Source: three-view drawing plus pictorial views. Frame: mm from the lowest corner of the part. A direction names the side the tool comes from. Coordinates: 2 decimals unless noted, no trailing zeros. Write each loop counter-clockwise with the first axis right and the second up, starting at its lowest first coordinate (ties: lowest second). Pieces come first, ordered by that corner, then holes. Notation, with made-up numbers: M 43,52 L 58,52 A34 ccw 58,84 Z; hole C 46,62 d10. An arc over 180 degrees is marked long. Write item = value, one per line. Start each with the question number.
Item 1: Ray query, L1, parallel to X at y = 1, z = 19; L2, parallel to Y at x = 18, z = 0.85; L3, parallel to X at y = 37.5, z = 2.8 (1 decimal). Return the intervals inside material, ascending. Write a range as [from, to].
Item 2: Section A-A on z = 19. Output: boundary loops of the cut face in (x, y).
Item 3: First-contact query: pin 1 Ø10 at (y, z) = (39, 7.5) entering from -X; pin 2 Ø5 at (x, y) = (18, 15) entering from +Z; pin 3 Ø8 at (x, z) = (30, 26) entering from +Y. Flat tips, straight axial feed; report the tip coordinate or a pass-through.
Item 4: Section B-B on y = 15. Output: boundary loops of the cut face in (x, z), plus the area to 3 significant figures.
Item 5: Section D-D on x = 23.5. Output: boundary loops of the cut face in (y, z), plus the area to 3 significant figures.
Item 6: Section C-C on x = 18. Output: boundary loops of the cut face in (y, z).
Item 7: Pull-direction query (X, two-part tool) for the marked faces 3, 4 and 5; classes: +X half, -X half, draft (parallel to the pull), parting line (faces both ways), or undercut.
Item 8: Reachability of the marked faces 1 and 2 from +Z, -Z, +X, -X, +Y, -Y: full face, straight path, thin tool, end or side. Return the list, or none.
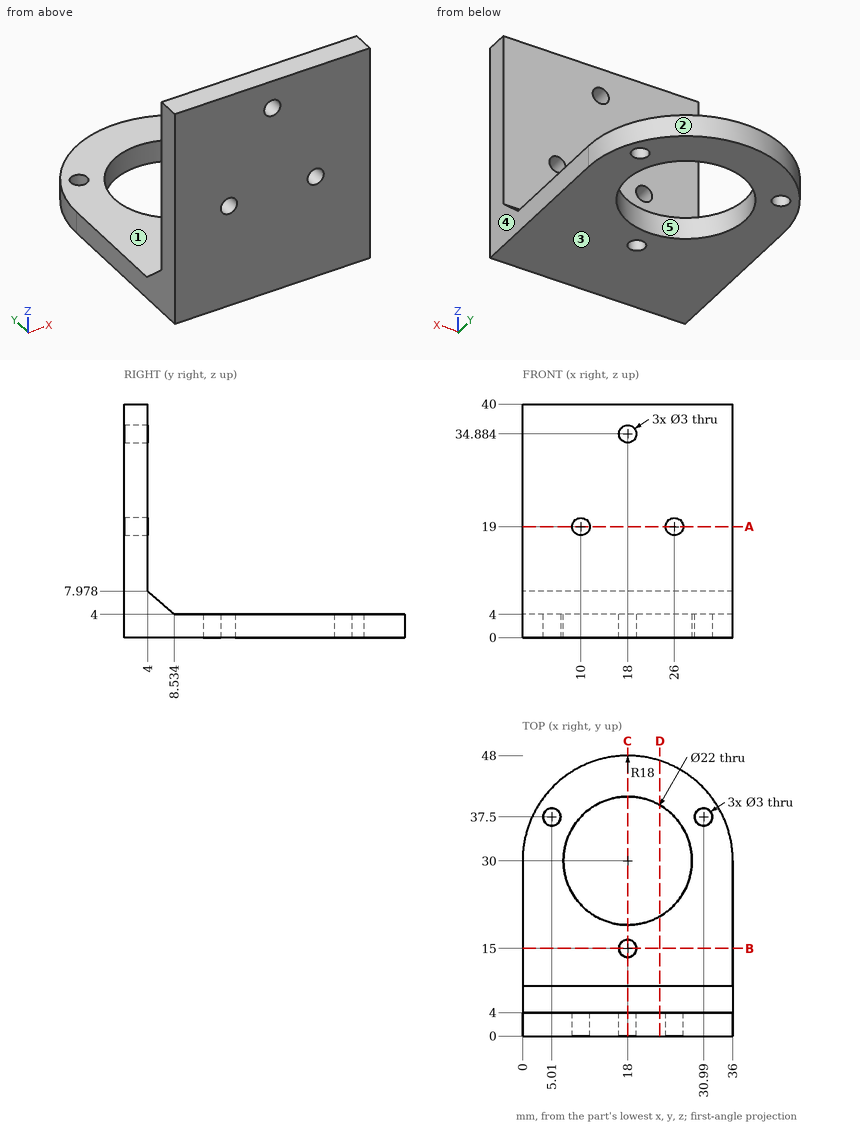
Responses:
q1.L1 = [0, 8.5], [11.5, 24.5], [27.5, 36]
q1.L2 = [0, 13.5], [16.5, 19], [41, 48]
q1.L3 = [1.6, 3.5], [6.5, 10], [26, 29.5], [32.5, 34.4]
q2.outline = M 0,0 L 8.5,0 L 8.5,4 L 0,4 Z; M 11.5,0 L 24.5,0 L 24.5,4 L 11.5,4 Z; M 27.5,0 L 36,0 L 36,4 L 27.5,4 Z
q3.pin_1 = 0.84
q3.pin_2 = 4
q3.pin_3 = 4
q4.outline = M 0,0 L 16.5,0 L 16.5,4 L 0,4 Z; M 19.5,0 L 36,0 L 36,4 L 19.5,4 Z
q4.area = 132 mm²
q5.outline = M 0,0 L 20.47,0 L 20.47,4 L 8.53,4 L 4,7.98 L 4,40 L 0,40 Z; M 39.53,0 L 47.14,0 L 47.14,4 L 39.53,4 Z
q5.area = 265 mm²
q6.outline = M 0,0 L 13.5,0 L 13.5,4 L 8.53,4 L 4,7.98 L 4,33.38 L 0,33.38 Z; M 0,36.38 L 4,36.38 L 4,40 L 0,40 Z; M 16.5,0 L 19,0 L 19,4 L 16.5,4 Z; M 41,0 L 48,0 L 48,4 L 41,4 Z
q7.face_3 = draft
q7.face_4 = +X half
q7.face_5 = undercut
q8.face_1 = +Z, +X, -X, +Y
q8.face_2 = +Z, -Z, +Y
